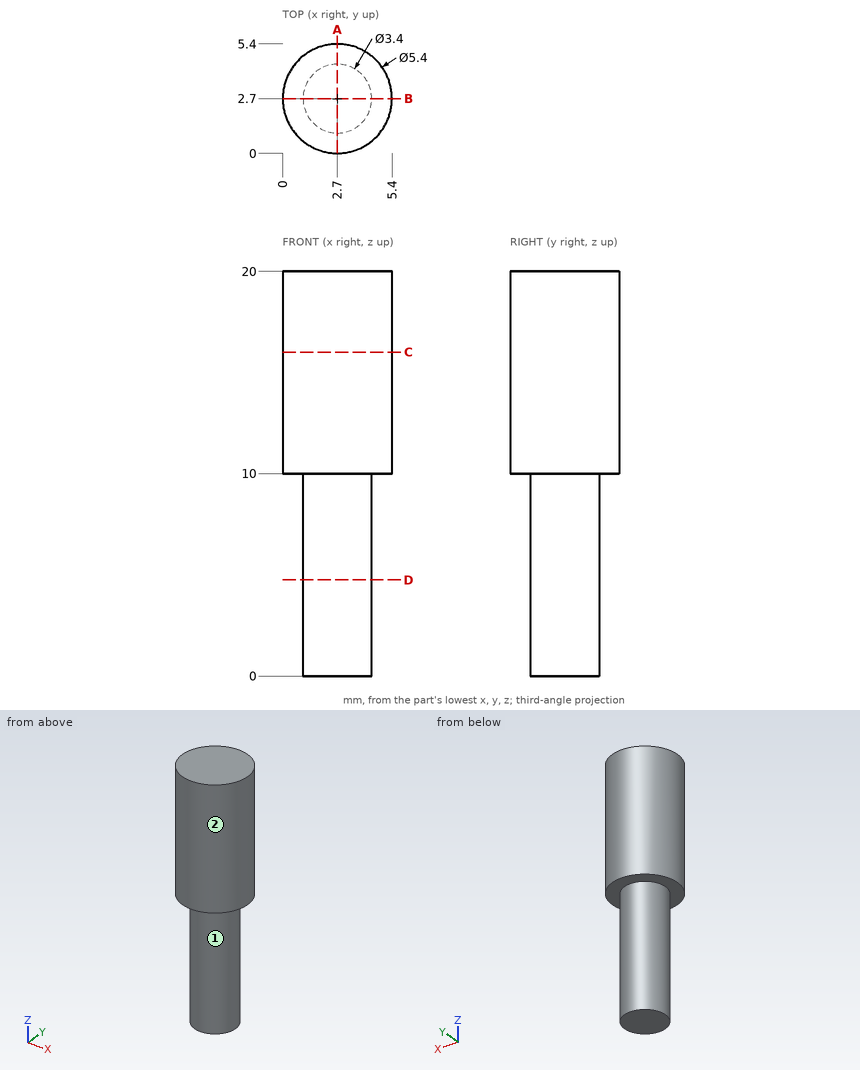
Could you check a few things on this drawing? It's one solid part, dimensions in mm from its lowest x, y, z. A direction names the side the tool comes from. Round coordinates to 2 decimals unless told otherwise and drop trailing zeros. Loops run counter-clockwise (first coordinate to the right, second up) from the corner with the lowest first, then second, coordinate; pieces in that order, holes last.
Q1. For P1, Ø1.6, axis at x = 2, y = 3, coming from the -Z side; P2, Ø2, axis at x = 1.5, z = 16, coming from the -Y side; P3, Ø3, axis at x = 4.5, z = 7, coming from the +Y side, each with a flat end and sliding along its axis, tell me the tip position at first contact or that it passes through.
Q2. I want a section at A-A (x = 2.7). Write out the boundary of the cut face in (y, z), and give its area (3 significant figures).
Q3. Please list where these lines run through material, in increasing order: L1, parallel to Z at x = 0.6, y = 1.95; L2, parallel to Y at x = 4.25, z = 8.75; L3, parallel to X at y = 4.05, z = 6.75.
Q4. I want a section at C-C (z = 16). Write out the boundary of the cut face in (x, y).
Q5. I want a section at D-D (z = 4.75). Write out the boundary of the cut face in (x, y), and give its area (3 significant figures).
Q6. On a 3-axis mill with a long thin cutter (end or side, diameter ignored), from which of +Z, -Z, +X, -X, +Y, -Y can I reach the whole of each face in a straight line? I mean the marked faces 1 and 2. Say none if no direction works.
Answer below:
1. P1: stops at z = 0
1. P2: stops at y = 0.01
1. P3: stops at y = 4.37
2. outline: (0, 10) - (1, 10) - (1, 0) - (4.4, 0) - (4.4, 10) - (5.4, 10) - (5.4, 20) - (0, 20) - close
2. area: 88.0 mm2
3. L1: z = 10 to 20
3. L2: y = 2 to 3.4
3. L3: x = 1.67 to 3.73
4. outline: circle Ø5.4 at (2.7, 2.7)
5. outline: circle Ø3.4 at (2.7, 2.7)
5. area: 9.08 mm2
6. face 1: -Z
6. face 2: +Z, -Z
